Part model, mm, in its own coordinate system. A direction names the side the tool comes from. Give positions to 0.01 mm unless a question says otherwise; leave off trailing zeros. Loops run counter-clockwise (first coordinate to the right, second up) from the corner with the lowest first, then second, coordinate; pieces in that order, holes last. Notation, with made-up numbers: M 88,-34.75 L 133,-34.75 A24 cw 133,-22.75 Z; hole C 58,68.25 d1. An arc over 180 degrees is marked long. Put each result on its own line as item: value. Start each with the question number.
```python
from build123d import *

# Parameters (mm, degrees)
SKETCH1_W             = 54
SKETCH1_H             = 27
SKETCH1_R             = 4
BOSS_EXTRUDE1_DEPTH   = 28
F_6_32_TAPPED_HOLE1_D = 2.7051
SKETCH4_W             = 16
SKETCH4_H             = 8
CUT_EXTRUDE1_DEPTH    = 55
CHAMFER1_SIZE         = 1


with BuildPart() as part:
    # Sketch1 → Boss-Extrude1 (new body)
    with BuildSketch(Plane(origin=(0, 0, 0), x_dir=(0, 0, -1), z_dir=(1, 0, 0))):
        with Locations((13, 0)):
            Rectangle(SKETCH1_W, SKETCH1_H)
        Circle(SKETCH1_R, mode=Mode.SUBTRACT)
    extrude(amount=-BOSS_EXTRUDE1_DEPTH)

    # #6-32 Tapped Hole1 (through all)
    with Locations(Plane(origin=(0, 0, 0), x_dir=(0, 0, -1), z_dir=(1, 0, 0))):
        with Locations((-8, 8), (-8, -8), (32, -8), (32, 8)):
            Hole(F_6_32_TAPPED_HOLE1_D / 2)

    # Sketch4 → Cut-Extrude1 (cut, through all)
    with BuildSketch(Plane.XY.offset(14)):
        with Locations((-14, 9.5)):
            Rectangle(SKETCH4_W, SKETCH4_H)
        with Locations((-14, -9.5)):
            Rectangle(SKETCH4_W, SKETCH4_H)
    extrude(amount=-CUT_EXTRUDE1_DEPTH, mode=Mode.SUBTRACT)

    # Chamfer1
    chamfer1_edges = [part.edges().sort_by_distance(p)[0] for p in [
        (-3, 13.5, -40),
        (-3, 13.5, 14),
        (-3, -13.5, 14),
        (-3, -13.5, -40),
        (-25, 13.5, 14),
        (-25, 13.5, -40),
        (-25, -13.5, -40),
        (-25, -13.5, 14),
    ]]
    chamfer(chamfer1_edges, length=CHAMFER1_SIZE)


solid = part.part
```
1) Pin check, flat tip, straight feed: pin 1 Ø13 at (x, z) = (-14, -7.5) entering from +Y. Stop position of the tip, or through.
2) Band-saw the part on A-A on y = 10. Give the cut face in (x, z).
3) Band-saw the part on D-D on x = -4.5. Give the cut face in (y, z).
4) Band-saw the part on C-C on z = 8. Give the cut face in (x, y).
5) Wall check: L1, parallel to Y at x = -2.75, z = -32; L2, parallel to X at y = 9.5, z = 2; L3, parallel to Y at x = -19.5, z = 0. Give the ranges that are in metal, low to high.
6) Mould opens along Z. For faces 4 (the flat face through (-14, 0, -40)), 5 (the cylindrical face through (-25.04, 8.41, -30.71)), 6 (the cylindrical face through (-3.04, -7.59, -30.71)), 7 (the flat face through (0, 0, -13)) say: +Z half, -Z half, draft (parallel to the pull), parting line (faces both ways), or undercut.
7) Band-saw the part on B-B on z = 0. Give the cut face in (x, y).
8) Which spindle directions (+Z, -Z, +X, -X, +Y, -Y) get a long thin tool onto all of the face, cutting with end or side? Do faces 1 (the cylindrical face through (-13.804, -3.905, 0.867)), 2 (the flat face through (-6, 9, -13)), 3 (the flat face through (-6, -10, -13)). Say none if no direction does.
Evaluation:
1. pin 1: y = 5.5
2. outline: M -28,-40 L -22,-40 L -22,14 L -28,14 Z; M -6,-40 L 0,-40 L 0,14 L -6,14 Z
3. outline: M -13.5,-39 L -12.5,-40 L 12.5,-40 L 13.5,-39 L 13.5,13 L 12.5,14 L -12.5,14 L -13.5,13 Z; hole C -8,-32 d2.71; hole C -8,8 d2.71; hole C 0,0 d8; hole C 8,-32 d2.71; hole C 8,8 d2.71
4. outline: M -28,-13.5 L -22,-13.5 L -22,-9.35 L -28,-9.35 Z; M -28,-6.65 L -22,-6.65 L -22,-5.5 L -6,-5.5 L -6,-6.65 L 0,-6.65 L 0,6.65 L -6,6.65 L -6,5.5 L -22,5.5 L -22,6.65 L -28,6.65 Z; M -28,9.35 L -22,9.35 L -22,13.5 L -28,13.5 Z; M -6,-13.5 L 0,-13.5 L 0,-9.35 L -6,-9.35 Z; M -6,9.35 L 0,9.35 L 0,13.5 L -6,13.5 Z
5. L1: -13.5 to -9.35, -6.65 to 6.65, 9.35 to 13.5
5. L2: -28 to -22, -6 to 0
5. L3: -5.5 to -4, 4 to 5.5
6. face 4: -Z half
6. face 5: undercut
6. face 6: undercut
6. face 7: draft
7. outline: M -28,-13.5 L -22,-13.5 L -22,-5.5 L -6,-5.5 L -6,-13.5 L 0,-13.5 L 0,-4 L -28,-4 Z; M -28,4 L 0,4 L 0,13.5 L -6,13.5 L -6,5.5 L -22,5.5 L -22,13.5 L -28,13.5 Z
8. face 1: +X, -X
8. face 2: +Z, -Z, +Y
8. face 3: +Z, -Z, -Y
